For this review, take the finished solid that the model builds, in its own axes (mm). Give positions to 0.01 mm unless a question says otherwise; leave off trailing zeros. Use one line per item in the form item = value. Start each with the question number.
Q1. Clearance check with flat-ended pins moving along their axes: pin 1 Ø1 at (y, z) = (2, 1.5) entering from -X; pin 2 Ø1.5 at (x, y) = (-6, 1.5) entering from -Z. State where each tip first meets the part, or that it passes through.
Q2. For probe 1 along Z at (x, y) = (-2, 0.75); probe 2 along Z at (x, y) = (-27.5, 0.7); probe 3 along Z at (x, y) = (1, 1.2), list the stretches that pass through material, from the lowest coordinate up. Write a range as [from, to].
Q3. Consider section A-A on z = -12. Give the number of separate pieces and of enclosed holes in the cut face, and give its area (3 significant figures).
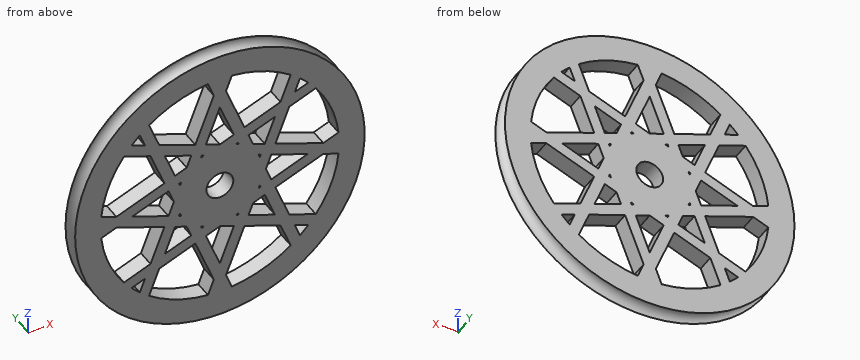
```python
from build123d import *

# Parameters (mm, degrees)
SKETCH2_R           = 8
SKETCH2_R_2         = 2.5
BOSS_EXTRUDE1_DEPTH = 3.175
BOSS_EXTRUDE2_START = -3.175
BOSS_EXTRUDE2_DEPTH = 3.175


with BuildPart() as part:
    # Sketch1 → Revolve2 (revolve)
    with BuildSketch(Plane.XY, mode=Mode.PRIVATE) as revolve2_sk:
        with BuildLine():
            Line((0, 0), (0, 3.175))
            Line((0, 3.175), (3.175, 3.175))
            Line((3.175, 3.175), (4.7625, 3.175))
            ThreePointArc((4.7625, 3.175), (3.175, 1.5875), (4.7625, 0))
            Line((4.7625, 0), (3.175, 0))
            Line((3.175, 0), (0, 0))
        make_face()
    revolve(revolve2_sk.sketch.rotate(Axis((-22.225, 12.769143385, 0), (0, -1, 0)), 180), axis=Axis((-22.225, 12.769143385, 0), (0, -1, 0)))



with BuildPart() as body_2:
    # Sketch2 → Boss-Extrude1 (new body)
    with BuildSketch(Plane(origin=(0, 0, 0), x_dir=(1, 0, 0), z_dir=(0, 1, 0))):
        with Locations(Location((-22.225, 0, 0), (0, 0, 180))):
            Circle(SKETCH2_R)
        with Locations(Location((-22.225, 0, 0), (0, 0, 180))):
            Circle(SKETCH2_R_2, mode=Mode.SUBTRACT)
    extrude(amount=BOSS_EXTRUDE1_DEPTH)


with BuildPart() as part_1:
    add(part.part)

    add(body_2.part)  # Boss-Extrude2 merges body 2
    # Sketch4 → Boss-Extrude2 (add)
    with BuildSketch(Plane.XZ.offset(BOSS_EXTRUDE2_START)):
        with BuildLine():
            Line((-22.224995499, -16.344642731), (-35.42857082, 17.877817054))
            ThreePointArc((-35.42857082, 17.877817054), (-36.308247437, 17.19339311), (-37.152505221, 16.465728434))
            Line((-37.152505221, 16.465728434), (-23.359368534, -19.284820497))
            Line((-23.359368534, -19.284820497), (-24.450638712, -22.113280112))
            ThreePointArc((-24.450638712, -22.113280112), (-22.225000553, -22.225), (-19.999362388, -22.113280223))
            Line((-19.999362388, -22.113280223), (-21.090626965, -19.284822234))
            Line((-21.090626965, -19.284822234), (-7.297444367, 16.465682732))
            ThreePointArc((-7.297444367, 16.465682732), (-8.141700351, 17.193350342), (-9.021375334, 17.877777286))
            Line((-9.021375334, 17.877777286), (-22.224995499, -16.344642731))
        make_face()
        with BuildLine():
            Line((-41.509820497, 1.134368534), (-5.759271566, 14.927505221))
            ThreePointArc((-5.759271566, 14.927505221), (-5.03160689, 14.083247437), (-4.347182946, 13.20357082))
            Line((-4.347182946, 13.20357082), (-38.569642731, -4.501e-06))
            Line((-38.569642731, -4.501e-06), (-4.347222714, -13.203624666))
            ThreePointArc((-4.347222714, -13.203624666), (-5.031649658, -14.083299649), (-5.759317268, -14.927555633))
            Line((-5.759317268, -14.927555633), (-41.509822234, -1.134373035))
            Line((-41.509822234, -1.134373035), (-44.338280223, -2.225637612))
            ThreePointArc((-44.338280223, -2.225637612), (-44.45, 5.53e-07), (-44.338280112, 2.225638712))
            Line((-44.338280112, 2.225638712), (-41.509820497, 1.134368534))
        make_face()
        with BuildLine():
            Line((-21.090631466, 19.284820497), (-7.297494779, -16.465728434))
            ThreePointArc((-7.297494779, -16.465728434), (-8.141752563, -17.19339311), (-9.02142918, -17.877817054))
            Line((-9.02142918, -17.877817054), (-22.225004501, 16.344642731))
            Line((-22.225004501, 16.344642731), (-35.428624666, -17.877777286))
            ThreePointArc((-35.428624666, -17.877777286), (-36.308299649, -17.193350342), (-37.152555633, -16.465682732))
            Line((-37.152555633, -16.465682732), (-23.359373035, 19.284822234))
            Line((-23.359373035, 19.284822234), (-24.450637612, 22.113280223))
            ThreePointArc((-24.450637612, 22.113280223), (-22.224999447, 22.225), (-19.999361288, 22.113280112))
            Line((-19.999361288, 22.113280112), (-21.090631466, 19.284820497))
        make_face()
        with BuildLine():
            Line((-2.940179503, -1.134368534), (-38.690728434, -14.927505221))
            ThreePointArc((-38.690728434, -14.927505221), (-39.41839311, -14.083247437), (-40.102817054, -13.20357082))
            Line((-40.102817054, -13.20357082), (-5.880357269, 4.501e-06))
            Line((-5.880357269, 4.501e-06), (-40.102777286, 13.203624666))
            ThreePointArc((-40.102777286, 13.203624666), (-39.418350342, 14.083299649), (-38.690682732, 14.927555633))
            Line((-38.690682732, 14.927555633), (-2.940177766, 1.134373035))
            Line((-2.940177766, 1.134373035), (-0.111719777, 2.225637612))
            ThreePointArc((-0.111719777, 2.225637612), (0, -5.53e-07), (-0.111719888, -2.225638712))
            Line((-0.111719888, -2.225638712), (-2.940179503, -1.134368534))
        make_face()
    extrude(amount=BOSS_EXTRUDE2_DEPTH)


solid = part_1.part
```
Working result:
q1.pin_1 = -47.87
q1.pin_2 = -20.15
q2.probe_1 = [-15.76, -9.21], [-1.5, 1.5], [9.21, 15.76]
q2.probe_2 = [-25.12, -21.59], [-10.61, 10.61], [21.59, 25.12]
q2.probe_3 = [-10.4, 10.4]
q3.separate_pieces = 6
q3.enclosed_holes = 0
q3.area = 77.6 mm²
